For this review, take the finished solid that the model builds, in its own axes (mm). Face numbers are marked on the shaded views. A direction names the side the tool comes from. Give positions to 0.01 mm unless a question says otherwise; leave off trailing zeros. Loops run counter-clockwise (first coordinate to the right, second up) from the corner with the lowest first, then second, coordinate; pieces in that order, holes last. Notation, with made-up numbers: (20.5, -32) - (24.5, -32) arc R18 ccw to (24.5, -11) - close; hole circle Ø5 at (-12, 87). An arc over 180 degrees is marked (long way). Put each result on its own line as item: value.
from build123d import *

# Parameters (mm, degrees)
F0_W          = 100
F0_H          = 80
F0_R          = 15
F1_DEPTH      = 50
F2_W          = 100
F2_H          = 30
F3_DEPTH      = 50.001
F3_DEPTH_BACK = 105.8
F4_R          = 10
F5_DEPTH      = 23.4


with BuildPart() as f1:
    # F0 (on Top) → F1 (new body)
    with BuildSketch(Plane.XY):
        Rectangle(F0_W, F0_H)
        Circle(F0_R, mode=Mode.SUBTRACT)
    extrude(amount=F1_DEPTH)

    # F2 (on Right) → F3 (cut, two sides)
    with BuildSketch(Plane.YZ) as f3_sk:
        with Locations((-35, 33.171409)):
            Rectangle(F2_W, F2_H)
    extrude(amount=F3_DEPTH, mode=Mode.SUBTRACT)
    extrude(f3_sk.sketch, amount=-F3_DEPTH_BACK, mode=Mode.SUBTRACT)

    # F4 (on Top) → F5 (cut)
    with BuildSketch(Plane.XY):
        with Locations((-27.791176, -23.038651)):
            Circle(F4_R)
        with Locations((31.747535, -21.252491)):
            Circle(F4_R)
    extrude(amount=F5_DEPTH, mode=Mode.SUBTRACT)


solid = f1.part
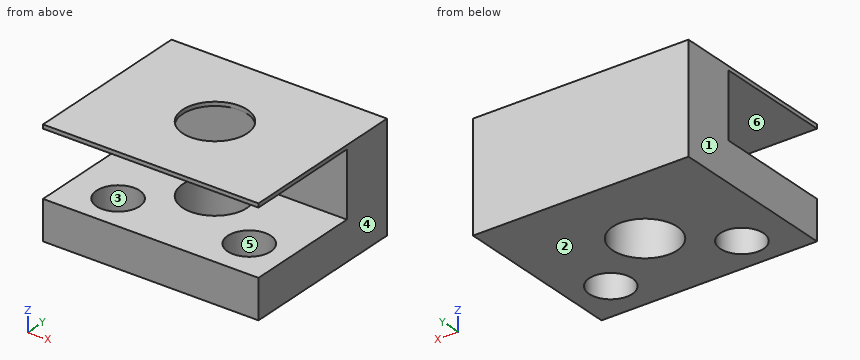
1) Take a section at D-D on x = 29. State the section outline as (y, z) points, and give its area (3 significant figures).
Geometry check:
outline: (-40, 0) - (-30.87, 0) - (-30.87, 18.17) - (-40, 18.17) - close; (-40, 48.17) - (15, 48.17) - (15, 18.17) - (-11.64, 18.17) - (-11.64, 0) - (40, 0) - (40, 50) - (-40, 50) - close
area: 2,000 mm²
2) Draft analysis for pull direction X (two halves, no side actions). For the marked faces 1, 2 and 3, state which applies: pulls with the +X half, pulls with the -X half, needs draft (parallel to the pull), parting line crosses it, or undercut.
Geometry check:
face 1: pulls with the -X half
face 2: needs draft
face 3: undercut
3) Insertion check: pin 1 Ø9 at (x, z) = (8, 39.5) entering from -Y; pin 2 Ø24 at (x, y) = (0, 0) entering from -Z. Each pin has a flat end and moves straight along its axis. Give the tip position at first contact, or say it passes through.
Geometry check:
pin 1: stops at y = 15
pin 2: passes through
4) For the marked faces 4, 5 and 6, list the 3-axis set-ups (+Z, -Z, +X, -X, +Y, -Y) from which the entire face can be reached by the end or side of a thin tool; tool diameter is ignored.
Geometry check:
face 4: +Z, -Z, +X, +Y, -Y
face 5: -Z
face 6: +X, -X, -Y
5) Wall thickness on line 1 (Z direction, x = -13.5, y = -26); line 2 (Y direction, x = 0, z = 49); line 3 (Y direction, x = 11, z = 38.5): over which ranges is each line inside the solid? List them lowest first.
Geometry check:
line 1: z = 0 to 18.17, 48.17 to 50
line 2: y = -40 to -15, 15 to 40
line 3: y = 15 to 40
6) Take a section at C-C on z = 8. State the section outline as (x, y) points, and give its area (3 significant figures).
Geometry check:
outline: (-50, -40) - (50, -40) - (50, 40) - (-50, 40) - close; hole circle Ø20 at (-27.79, -23.04); hole circle Ø30 at (0, 0); hole circle Ø20 at (31.75, -21.25)
area: 6,660 mm²
7) Take a section at A-A on y = 0. State the section outline as (x, z) points, and give its area (3 significant figures).
Geometry check:
outline: (-50, 0) - (-15, 0) - (-15, 18.17) - (-50, 18.17) - close; (-50, 48.17) - (-15, 48.17) - (-15, 50) - (-50, 50) - close; (15, 0) - (50, 0) - (50, 18.17) - (15, 18.17) - close; (15, 48.17) - (50, 48.17) - (50, 50) - (15, 50) - close
area: 1,400 mm²
8) Take a section at B-B on x = -8.5. State the section outline as (y, z) points.
Geometry check:
outline: (-40, 0) - (-12.36, 0) - (-12.36, 18.17) - (-40, 18.17) - close; (-40, 48.17) - (-12.36, 48.17) - (-12.36, 50) - (-40, 50) - close; (12.36, 0) - (40, 0) - (40, 50) - (12.36, 50) - (12.36, 48.17) - (15, 48.17) - (15, 18.17) - (12.36, 18.17) - close
